Verification items for the finished model (mm, model axes). A direction names the side the tool comes from. Round coordinates to 2 decimals unless told otherwise and drop trailing zeros. Loops run counter-clockwise (first coordinate to the right, second up) from the corner with the lowest first, then second, coordinate; pieces in that order, holes last. Notation, with made-up numbers: M 59.25,24 L 67.25,24 A21 ccw 67.25,38 Z; hole C 82,7 d6. An arc over 180 degrees is marked long. Answer as CSV lines item,"result".
```python
from build123d import *

# Parameters (mm, degrees)
SKETCH_1_R          = 14.85
EXTRUDE_1_DEPTH     = 13
SKETCH_2_R          = 10
EXTRUDE_2_DEPTH     = 17
CUT_EXTRUDE_1_DEPTH = 12
SKETCH_13_R         = 1.4
CUT_EXTRUDE_2_DEPTH = 13.25


with BuildPart() as part:
    # 스케치1 → 보스-돌출1 (new body)
    with BuildSketch(Plane(origin=(0, 0, 0), x_dir=(1, 0, 0), z_dir=(0, 1, 0))):
        Circle(SKETCH_1_R)
    extrude(amount=EXTRUDE_1_DEPTH)

    # 스케치2 → 보스-돌출2 (add)
    with BuildSketch(Plane(origin=(0, 13, 0), x_dir=(1, 0, 0), z_dir=(0, 1, 0))):
        Circle(SKETCH_2_R)
    extrude(amount=EXTRUDE_2_DEPTH)

    # 스케치4 → 컷-돌출1 (cut)
    with BuildSketch(Plane(origin=(0, 30, 0), x_dir=(1, 0, 0), z_dir=(0, 1, 0))):
        with BuildLine():
            Line((-1.688194302, -2.6), (1.688194302, -2.6))
            ThreePointArc((1.688194302, -2.6), (0, 3.1), (-1.688194302, -2.6))
        make_face()
    extrude(amount=-CUT_EXTRUDE_1_DEPTH, mode=Mode.SUBTRACT)

    # 스케치13 → 컷-돌출2 (cut, through all)
    with BuildSketch(Plane(origin=(0, 0, 2.6), x_dir=(-1, 0, 0), z_dir=(0, 0, -1))):
        with Locations((0, 24)):
            Circle(SKETCH_13_R)
    extrude(amount=-CUT_EXTRUDE_2_DEPTH, mode=Mode.SUBTRACT)

    # 스케치3 → 회전1 (revolve)
    with BuildSketch(Plane(origin=(0, 0, 0), x_dir=(0, 0, -1), z_dir=(1, 0, 0))):
        with BuildLine():
            ThreePointArc((-14.85, 13), (-11.420532111, 14.420532111), (-10, 17.85))
            Line((-10, 17.85), (-10, 13))
            Line((-10, 13), (-14.85, 13))
        make_face()
    revolve(axis=Axis((0, 34.691748642, 0), (0, -1, 0)))


solid = part.part
```
1) Section check A-A (x = 0). Record the cut outline in (y, z).
Here are the results:
outline,"M 0,-14.85 L 13,-14.85 A4.85 cw 17.85,-10 L 30,-10 L 30,-3.1 L 18,-3.1 L 18,2.6 L 22.6,2.6 L 22.6,10 L 17.85,10 A4.85 cw 13,14.85 L 0,14.85 Z; M 25.4,2.6 L 30,2.6 L 30,10 L 25.4,10 Z"
2) Section check B-B (z = 0). Record the cut outline in (x, y).
Here are the results:
outline,"M -14.85,0 L 14.85,0 L 14.85,13 A4.85 cw 10,17.85 L 10,30 L 3.1,30 L 3.1,18 L -3.1,18 L -3.1,30 L -10,30 L -10,17.85 A4.85 cw -14.85,13 Z"
3) Section check D-D (y = 6). Record the cut outline in (x, z).
Here are the results:
outline,"C 0,0 d29.7"
4) Draft check along Z on faces 1 (the flat face through (0, 18, 0)), 2 (the flat face through (-0.8, 25.4, 2.6)), 3 (the cylindrical face through (9.54, 23.84, -3)), 4 (the flat face through (0, 0, 0)). Enter one of: +Z half, -Z half, draft (parallel to the pull), parting line (faces both ways), or undercut.
Here are the results:
face 1,"undercut"
face 2,"undercut"
face 3,"parting line"
face 4,"draft"
5) Set-up check for faces 5 (the cylindrical face through (0.1, 24.1, -3.1)), 6 (the cylindrical face through (0.303, 22.633, 6.25)), 7 (the flat face through (-2.4, 30, -2.4)): record each of +Z, -Z, +X, -X, +Y, -Y from which the full face is reachable in a straight line by a thin tool's end or side.
Here are the results:
face 5,"+Y"
face 6,"+Z"
face 7,"+Z, -Z, +X, -X, +Y"
6) Go/stop test with flat-tipped pins: pin 1 (5 mm diameter, centred on x = 10.5, y = 20.5, fed in from -Z); pin 2 (3 mm diameter, centred on y = 13, z = 0.5, fed in from -X); pin 3 (1 mm diameter, centred on x = 0, y = 23, fed in from -Z); pin 4 (12 mm diameter, centred on y = 7, z = 11.5, fed in from +X). Record where each tip stops, or that it passes through.
Here are the results:
pin 1,"stops at z = -6"
pin 2,"stops at x = -14.85"
pin 3,"stops at z = -10"
pin 4,"stops at x = 13.79"
7) Section check C-C (y = 24). Record the cut outline in (x, z), plus the area to 3 significant figures.
Here are the results:
outline,"M -1.69,2.6 L -1.4,2.6 L -1.4,9.9 A10 ccw long 1.4,9.9 L 1.4,2.6 L 1.69,2.6 A3.1 cw long Z"
area,"264 mm^2"
8) Material ranges on probe 1 along Y at (x, z) = (0, 5.5); probe 2 along Z at (x, y) = (0, 21.5); probe 3 along X at (y, z) = (29, 1.5), recorded low to high.
Here are the results:
probe 1,"y = 0 to 22.6, 25.4 to 30"
probe 2,"z = -10 to -3.1, 2.6 to 10"
probe 3,"x = -9.89 to -2.71, 2.71 to 9.89"
